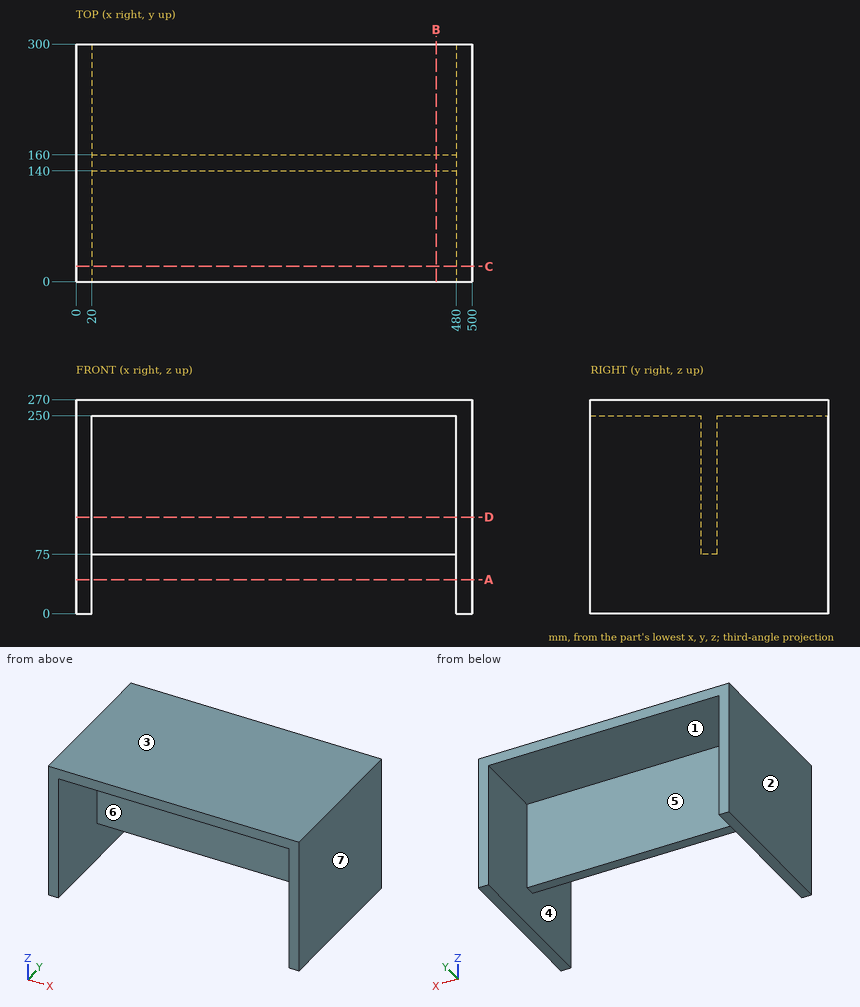
Study the drawing (mm; zero at the part's minimum x, y, z) and answer. A direction names the side the tool comes from. Coordinates: 2 decimals unless noted, no trailing zeros. Order: outer loops, then holes, each group sorted by start corner. A loop starts at its lowest first (then second) coordinate and runs counter-clockwise, first axis right, second up. Notation, with made-up numbers: M -4,88.25 L 5,88.25 A14 ccw 5,95.25 Z; hole C -0.75,66 d6. An arc over 180 degrees is marked long. Answer as a JSON object with one key per item and string values. Group by question number.
1. Section B-B on x = 454.5 is taken. Write down the section's boundary in (y, z), then the cut area to 3 significant figures.
2. Determine the mould class of the marked faces 1, 2 and 3 for opening direction X: released by +X, released by -X, zero draft, split by the parting line, or undercut.
3. Flat-ended cylindrical pins translate along their axes: P1, Ø3, axis at x = 191.5, z = 82, coming from the +Y side; P2, Ø2, axis at y = 71, z = 223, coming from the -X side; P3, Ø12, axis at x = 111.5, y = 216.5, coming from the -Z side; P4, Ø8, axis at x = 185.5, z = 190, coming from the -Y side. Find the tip coordinate at first contact, or state that the pin passes through.
4. A tool of negligible diameter and unlimited length cuts with its end or side. For the marked faces 4, 5, 6 and 7, from which of +Z, -Z, +X, -X, +Y, -Y can it reach the whole face along a straight path? Write none if from no direction.
5. Straight lines are drawn through the part: line 1 (X direction, y = 62.5, z = 98); line 2 (Z direction, x = 312.5, y = 111); line 3 (Y direction, x = 96, z = 155). For each, find the intervals that lie inside material, in ascending order.
6. Section D-D on z = 122 is taken. Write down the section's boundary in (x, y).
7. Section C-C on y = 19.5 is taken. Write down the section's boundary in (x, z), then the cut area to 3 significant figures.
8. Section A-A on z = 43 is taken. Write down the section's boundary in (x, y).
Values follow:
{
 "1": {"outline": "M 0,250 L 140,250 L 140,75 L 160,75 L 160,250 L 300,250 L 300,270 L 0,270 Z", "area": "9,500 mm2"},
 "2": {"face 1": "undercut", "face 2": "released by -X", "face 3": "zero draft"},
 "3": {"P1": "y = 160", "P2": "x = 0", "P3": "z = 250", "P4": "y = 140"},
 "4": {"face 4": "-Z", "face 5": "-Z, +Y", "face 6": "-Z, -Y", "face 7": "+Z, -Z, +X, +Y, -Y"},
 "5": {"line 1": "0 to 20, 480 to 500", "line 2": "250 to 270", "line 3": "140 to 160"},
 "6": {"outline": "M 0,0 L 20,0 L 20,140 L 480,140 L 480,0 L 500,0 L 500,300 L 480,300 L 480,160 L 20,160 L 20,300 L 0,300 Z"},
 "7": {"outline": "M 0,0 L 20,0 L 20,250 L 480,250 L 480,0 L 500,0 L 500,270 L 0,270 Z", "area": "20,000 mm2"},
 "8": {"outline": "M 0,0 L 20,0 L 20,300 L 0,300 Z; M 480,0 L 500,0 L 500,300 L 480,300 Z"}
}
